```python
from build123d import *

# Parameters (mm, degrees)
ESQUISSE1_R        = 1.6
BOSS_EXTRU_1_DEPTH = 1.6
ESQUISSE2_W        = 9
ESQUISSE2_H        = 11
BOSS_EXTRU_2_DEPTH = 12.7
ESQUISSE3_R        = 6.25
BOSS_EXTRU_3_DEPTH = 22
ESQUISSE4_W        = 27.9
ESQUISSE4_H        = 19.8
BOSS_EXTRU_4_DEPTH = 19


with BuildPart() as part:
    # Esquisse1 → Boss.-Extru.1 (new body)
    with BuildSketch(Plane.XY):
        Polygon((0, 0), (80, 0), (80, -50), (60, -70), (0, -70), align=None)
        with Locations((17, -4)):
            Circle(ESQUISSE1_R, mode=Mode.SUBTRACT)
        with Locations((66, -4)):
            Circle(ESQUISSE1_R, mode=Mode.SUBTRACT)
        with Locations((58, -66)):
            Circle(ESQUISSE1_R, mode=Mode.SUBTRACT)
        with Locations((4, -66)):
            Circle(ESQUISSE1_R, mode=Mode.SUBTRACT)
    extrude(amount=BOSS_EXTRU_1_DEPTH)

    # Esquisse2 → Boss.-Extru.2 (add)
    with BuildSketch(Plane.XY.offset(1.6)):
        with Locations((4.5, -6.5)):
            Rectangle(ESQUISSE2_W, ESQUISSE2_H)
        with Locations((75.5, -6.5)):
            Rectangle(ESQUISSE2_W, ESQUISSE2_H)
        with Locations((75.5, -18.5)):
            Rectangle(ESQUISSE2_W, ESQUISSE2_H)
        with Locations((75.5, -30.5)):
            Rectangle(ESQUISSE2_W, ESQUISSE2_H)
        with Locations((75.5, -42.5)):
            Rectangle(ESQUISSE2_W, ESQUISSE2_H)
    extrude(amount=BOSS_EXTRU_2_DEPTH)

    # Esquisse3 → Boss.-Extru.3 (add)
    with BuildSketch(Plane.XY.offset(1.6)):
        with Locations(Location((8, -20, 0), (0, 0, 180))):
            Circle(ESQUISSE3_R)
        with Locations(Location((8, -33, 0), (0, 0, 180))):
            Circle(ESQUISSE3_R)
        with Locations(Location((8, -56, 0), (0, 0, 180))):
            Circle(ESQUISSE3_R)
        with Locations(Location((62, -20, 0), (0, 0, 180))):
            Circle(ESQUISSE3_R)
        with Locations(Location((62, -33, 0), (0, 0, 180))):
            Circle(ESQUISSE3_R)
    extrude(amount=BOSS_EXTRU_3_DEPTH)

    # Esquisse4 → Boss.-Extru.4 (add)
    with BuildSketch(Plane.XY.offset(1.6)):
        with Locations((35.95, -14.9)):
            Rectangle(ESQUISSE4_W, ESQUISSE4_H)
    extrude(amount=BOSS_EXTRU_4_DEPTH)


solid = part.part
```
Input: part model. Units: mm. Frame: model coordinates. A direction names the side the tool comes from. Coordinates: 2 decimals unless noted, no trailing zeros. Write each loop counter-clockwise with the first axis right and the second up, starting at its lowest first coordinate (ties: lowest second). Pieces come first, ordered by that corner, then holes.
1) Section B-B on y = -4. Output: boundary loops of the cut face in (x, z).
2) Pin query (flat end, axial travel): pin 1 Ø8 at (y, z) = (-51.5, 11.5) entering from -X; pin 2 Ø2.5 at (x, z) = (76.5, 7.5) entering from -Y; pin 3 Ø10 at (x, y) = (48, -59) entering from +Z; pin 4 Ø4 at (x, y) = (58, -66) entering from -Z. Return the tip coordinate at first contact, or that it passes through.
3) Mould query, pull axis X, two halves, no side actions, for faces 6 (the flat face through (22, -15, 11)), 7 (the flat face through (75, -48, 8)), 8 (the flat face through (0, -17, 1)). Classes: pulls with the +X half, pulls with the -X half, needs draft (parallel to the pull), parting line crosses it, or undercut.
4) Section D-D on z = 21.75. Output: boundary loops of the cut face in (x, y), and give its area (3 significant figures).
5) Set-up query: faces 1 (the flat face through (75, -13, 8)), 2 (the flat face through (4, -6, 14.3)), 3 (the flat face through (75, -42, 14.3)), 4 (the cylindrical face through (9.355, -13.899, 12.446)), 5 (the flat face through (49.9, -15, 11)). Return all of +Z, -Z, +X, -X, +Y, -Y with unobstructed straight access to the full face (end or side cutting, diameter ignored); none if empty.
6) Section A-A on x = 17. Output: boundary loops of the cut face in (y, z), and give its area (3 significant figures).
7) Material intervals for line 1 along Y through (x, z) = (75.5, 6); line 2 along Y through (x, z) = (17, 0.55); line 3 along X through (y, z) = (-66, 1.1), sorted ascending.
8) Section C-C on z = 12.75. State how many separate pieces and enclosed holes the cut face has, and give its area (3 significant figures).
Check result:
1. outline: (0, 0) - (15.4, 0) - (15.4, 1.6) - (9, 1.6) - (9, 14.3) - (0, 14.3) - close; (18.6, 0) - (64.4, 0) - (64.4, 1.6) - (18.6, 1.6) - close; (67.6, 0) - (80, 0) - (80, 14.3) - (71, 14.3) - (71, 1.6) - (67.6, 1.6) - close
2. pin 1: stops at x = 1.77
2. pin 2: stops at y = -48
2. pin 3: stops at z = 1.6
2. pin 4: stops at z = 0
3. face 6: undercut
3. face 7: needs draft
3. face 8: pulls with the -X half
4. outline: circle Ø12.5 at (8, -56); circle Ø12.5 at (8, -33); circle Ø12.5 at (8, -20); circle Ø12.5 at (62, -33); circle Ø12.5 at (62, -20)
4. area: 614 mm2
5. face 1: +Z, +X
5. face 2: +Z, -X, +Y
5. face 3: +Z, +X, +Y, -Y
5. face 4: +Z
5. face 5: +Z, +Y, -Y
6. outline: (-70, 0) - (-5.6, 0) - (-5.6, 1.6) - (-70, 1.6) - close; (-2.4, 0) - (0, 0) - (0, 1.6) - (-2.4, 1.6) - close
6. area: 107 mm2
7. line 1: y = -48 to -37, -36 to -25, -24 to -13, -12 to -1
7. line 2: y = -70 to -5.6, -2.4 to 0
7. line 3: x = 0 to 2.4, 5.6 to 56.4, 59.6 to 64
8. separate pieces: 11
8. enclosed holes: 0
8. area: 1,660 mm2
